Build history of the part. All positions in model axes, mm. A direction names the side the tool comes from. Give positions to 0.01 mm unless a question says otherwise; leave off trailing zeros. Loops run counter-clockwise (first coordinate to the right, second up) from the corner with the lowest first, then second, coordinate; pieces in that order, holes last. Notation, with made-up numbers: M -29,69 L -20,69 A22 cw -20,89 Z; hole C 42.5,5.25 d7. An arc over 180 degrees is marked long. Answer as a JSON object with one key per item and string values. Group by question number.
1. Slice it at B-B (z = 51). List the corners of the cut face in (x, y).
2. Slice it at C-C (x = 11.25). List the corners of the cut face in (y, z), then the cut area to 3 significant figures.
3. Mould opens along X. For faces 1 (the face through (6.431, 10, 30)), 2 (the face through (27, 17.659, 30)), 3 (the face through (32.931, 11, 30)), 4 (the face through (34.431, 10, 30)) say: released by +X, released by -X, zero draft, split by the parting line, or undercut.
4. Drill centre lines: line 1 along X through (y, z) = (8.25, 32); line 2 along Y through (x, z) = (31, 19.5). Where is each one in solid material? Low to high. Write a range as [from, to].
5. Drop a flat-ended pin along its axis: pin 1 Ø1.5 at (x, z) = (30, 44) entering from +Y. Give the stop position or say it passes through.
6. Slice it at A-A (y = 15). List the corners of the cut face in (x, z), then the cut area to 3 significant figures.
7. 3-axis set-ups, long thin cutter, end or side, ignore diameter. For faces 5 (the face through (21, 4.659, 30)), 6 (the face through (14, 17.659, 30)): which of +Z, -Z, +X, -X, +Y, -Y reach the whole face in a straight line?
from build123d import *

# Parameters (mm, degrees)
EXTRUDE_DEPTH                     = 60
EXTRUDE_ONTO_WIRE_PLACEMENT_ANGLE = 3.1e-05


with BuildPart() as part:
    # Wire as drawn → Extrude (new)
    with BuildSketch(Plane.XY):
        Polygon((0, 0), (28, 0), (28, 16), (26.5, 16), (26.5, 3), (21.5, 3), (21.5, 16), (20, 16), (20, 3), (8, 3), (8, 16), (6.5, 16), (6.5, 3), (1.5, 3), (1.5, 16), (0, 16), align=None)
    extrude(amount=EXTRUDE_DEPTH)


with BuildPart() as part_1:
    # Extrude onto Wire placement: moved
    add(part.part.moved(Location((6.431091, 1.659197, 0))).rotate(Axis((6.431091, 1.659197, 0), (0, 0, 1)), EXTRUDE_ONTO_WIRE_PLACEMENT_ANGLE))


solid = part_1.part
Established:
{
 "1": {"outline": "M 6.43,1.66 L 34.43,1.66 L 34.43,17.66 L 32.93,17.66 L 32.93,4.66 L 27.93,4.66 L 27.93,17.66 L 26.43,17.66 L 26.43,4.66 L 14.43,4.66 L 14.43,17.66 L 12.93,17.66 L 12.93,4.66 L 7.93,4.66 L 7.93,17.66 L 6.43,17.66 Z"},
 "2": {"outline": "M 1.66,0 L 4.66,0 L 4.66,60 L 1.66,60 Z", "area": "180 mm^2"},
 "3": {"face 1": "released by -X", "face 2": "zero draft", "face 3": "undercut", "face 4": "released by +X"},
 "4": {"line 1": "x = [6.43, 7.93], [12.93, 14.43], [26.43, 27.93], [32.93, 34.43]", "line 2": "y = [1.66, 4.66]"},
 "5": {"pin 1": "stops at y = 4.66"},
 "6": {"outline": "M 6.43,0 L 7.93,0 L 7.93,60 L 6.43,60 Z; M 12.93,0 L 14.43,0 L 14.43,60 L 12.93,60 Z; M 26.43,0 L 27.93,0 L 27.93,60 L 26.43,60 Z; M 32.93,0 L 34.43,0 L 34.43,60 L 32.93,60 Z", "area": "360 mm^2"},
 "7": {"face 5": "+Z, -Z, +Y", "face 6": "+Z, -Z, +X, -X, +Y"}
}
